For this review, take the finished solid that the model builds, in its own axes (mm). A direction names the side the tool comes from. Coordinates: 2 decimals unless noted, no trailing zeros. Loops run counter-clockwise (first coordinate to the right, second up) from the corner with the lowest first, then second, coordinate; pieces in that order, holes last. Notation, with made-up numbers: M 20,54 L 44,54 A22 cw 44,71 Z; hole C 12,34 d10. An arc over 180 degrees is marked long. Put each result on its own line as item: value.
```python
from build123d import *

# Parameters (mm, degrees)
SKETCH1_W           = 11.7
SKETCH1_H           = 4.8
BOSS_EXTRUDE1_DEPTH = 0.35
SKETCH2_W           = 4
SKETCH2_H           = 1
CUT_EXTRUDE2_DEPTH  = 0.3
BOSS_EXTRUDE3_DEPTH = 0.35
FILLET2_R           = 0.1
SKETCH6_W           = 0.5
SKETCH6_H           = 1
CUT_EXTRUDE3_DEPTH  = 1


with BuildPart() as part:
    # Sketch1 → Boss-Extrude1 (new body)
    with BuildSketch(Plane(origin=(0, 0, 0), x_dir=(1, 0, 0), z_dir=(0, 1, 0))):
        Rectangle(SKETCH1_W, SKETCH1_H)
    extrude(amount=BOSS_EXTRUDE1_DEPTH)

    # Sketch2 → Cut-Extrude2 (cut)
    with BuildSketch(Plane.XZ):
        with Locations((-3.85, 0)):
            Rectangle(SKETCH2_W, SKETCH2_H)
        with Locations((3.85, 0)):
            Rectangle(SKETCH2_W, SKETCH2_H)
    extrude(amount=-CUT_EXTRUDE2_DEPTH, mode=Mode.SUBTRACT)

    # Sketch4 → Boss-Extrude3 (add)
    with BuildSketch(Plane(origin=(0, 0.35, 0), x_dir=(1, 0, 0), z_dir=(0, 1, 0))):
        with BuildLine():
            Line((-4.35, 2.15), (-4.35, 2.4))
            Line((-4.35, 2.4), (-5.85, 2.4))
            Line((-5.85, 2.4), (-5.85, 0.9))
            Line((-5.85, 0.9), (-5.6, 0.9))
            ThreePointArc((-5.6, 0.9), (-5.107388458, 1.657388458), (-4.35, 2.15))
        make_face()
        with BuildLine():
            Line((5.85, 2.4), (4.35, 2.4))
            Line((4.35, 2.4), (4.35, 2.15))
            ThreePointArc((4.35, 2.15), (5.107388458, 1.657388458), (5.6, 0.9))
            Line((5.6, 0.9), (5.85, 0.9))
            Line((5.85, 0.9), (5.85, 2.4))
        make_face()
        with BuildLine():
            Line((4.35, -2.15), (4.35, -2.4))
            Line((4.35, -2.4), (5.85, -2.4))
            Line((5.85, -2.4), (5.85, -0.9))
            Line((5.85, -0.9), (5.6, -0.9))
            ThreePointArc((5.6, -0.9), (5.107388458, -1.657388458), (4.35, -2.15))
        make_face()
        with BuildLine():
            Line((-5.85, -2.4), (-4.35, -2.4))
            Line((-4.35, -2.4), (-4.35, -2.15))
            ThreePointArc((-4.35, -2.15), (-5.107388458, -1.657388458), (-5.6, -0.9))
            Line((-5.6, -0.9), (-5.85, -0.9))
            Line((-5.85, -0.9), (-5.85, -2.4))
        make_face()
    extrude(amount=BOSS_EXTRUDE3_DEPTH)

    # Fillet2
    fillet2_edges = [part.edges().sort_by_distance(p)[0] for p in [
        (5.85, 0.35, 2.4),
        (-5.85, 0.35, 2.4),
        (-5.85, 0.35, -2.4),
        (5.85, 0.35, -2.4),
    ]]
    fillet(fillet2_edges, radius=FILLET2_R)

    # Sketch6 → Cut-Extrude3 (cut)
    with BuildSketch(Plane.XZ.offset(-0.3)):
        with Locations((2.44, 0)):
            Rectangle(SKETCH6_W, SKETCH6_H)
        with Locations((-2.44, 0)):
            Rectangle(SKETCH6_W, SKETCH6_H)
    extrude(amount=-CUT_EXTRUDE3_DEPTH, mode=Mode.SUBTRACT)


solid = part.part
```
(1) Add section D-D (z = 1.45). Write out the cut boundary in (x, y).
Determined:
outline: M -5.85,0 L 5.85,0 L 5.85,0.7 L 5.29,0.7 L 5.29,0.35 L -5.29,0.35 L -5.29,0.7 L -5.85,0.7 Z
(2) Wall thickness on line 1 along Z through (x, y) = (3.25, 0.1); line 2 along Y through (x, z) = (-0.25, 1.25); line 3 along X through (y, z) = (0.4, -2): over which ranges is each line inside the solid? List them lowest first. Write a range as [from, to].
Determined:
line 1: z = [-2.4, -0.5], [0.5, 2.4]
line 2: y = [0, 0.35]
line 3: x = [-5.85, -4.66], [4.66, 5.85]
(3) Tool access review of faces 1 (the flat face through (-5, 0.7, 2)), 2 (the cylindrical face through (-5.116, 0.523, -1.648)): name each direction out of +Z, -Z, +X, -X, +Y, -Y from which nothing blocks a thin tool from reaching the whole face with its end or side.
Determined:
face 1: +Z, -Z, +X, -X, +Y
face 2: +Y
(4) Draft analysis for pull direction X (two halves, no side actions). For faces 3 (the flat face through (0, 0, 0)), 4 (the cylindrical face through (-5.098, 0.523, 1.666)), state which applies: +X half, -X half, draft (parallel to the pull), parting line (faces both ways), or undercut.
Determined:
face 3: draft
face 4: undercut
(5) Add section A-A (z = 0.25). Write out the cut boundary in (x, y).
Determined:
outline: M -5.85,0.3 L -2.69,0.3 L -2.69,0.35 L -5.85,0.35 Z; M -2.19,0.3 L -1.85,0.3 L -1.85,0 L 1.85,0 L 1.85,0.3 L 2.19,0.3 L 2.19,0.35 L -2.19,0.35 Z; M 2.69,0.3 L 5.85,0.3 L 5.85,0.35 L 2.69,0.35 Z
(6) Add section B-B (y = 0.55). Write out the cut boundary in (x, z).
Determined:
outline: M -5.85,-2.3 A0.1 ccw -5.75,-2.4 L -4.35,-2.4 L -4.35,-2.15 A2.18 cw -5.6,-0.9 L -5.85,-0.9 Z; M -5.85,0.9 L -5.6,0.9 A2.18 cw -4.35,2.15 L -4.35,2.4 L -5.75,2.4 A0.1 ccw -5.85,2.3 Z; M 4.35,-2.4 L 5.75,-2.4 A0.1 ccw 5.85,-2.3 L 5.85,-0.9 L 5.6,-0.9 A2.18 cw 4.35,-2.15 Z; M 4.35,2.15 A2.18 cw 5.6,0.9 L 5.85,0.9 L 5.85,2.3 A0.1 ccw 5.75,2.4 L 4.35,2.4 Z
(7) Add section C-C (x = -3.5). Write out the cut boundary in (y, z), plus the area to 3 significant figures.
Determined:
outline: M 0,-2.4 L 0.35,-2.4 L 0.35,2.4 L 0,2.4 L 0,0.5 L 0.3,0.5 L 0.3,-0.5 L 0,-0.5 Z
area: 1.38 mm^2
